from build123d import *

# Parameters (mm, degrees)
F1_DEPTH    = 6.35
F2_T1_DEPTH = 38.1
F2_T3_DEPTH = 33.8463065702
F4_DEPTH    = 6.351


# Not quite as in the source:
# - a fillet or chamfer that OpenCascade refuses, or shapes differently, is made with other operations: its cross-section is extruded or revolved along the edge and cut away or added


with BuildPart() as f1:
    # F0 (on Top) → F1 (new body)
    with BuildSketch(Plane.XY):
        Polygon((-3.1513119073, 592.2723904558), (-22.2013119073, 592.2723904558), (-22.2013119073, 439.8723904558), (-19.0263119073, 439.8723904558), (-19.0263119073, -68.1276095442), (-6.3263119073, -68.1276095442), (-6.3263119073, 439.8723904558), (-3.1513119073, 439.8723904558), align=None)
    extrude(amount=F1_DEPTH)

    # F2: fillet of radius 6.35 on 4 edges, made by hand

    # F2_s2 → F2_t1 (cut)
    with BuildSketch(Plane.XY.offset(-15.875)):
        with BuildLine():
            ThreePointArc((-3.1513119073, 585.9223904558), (-5.0111838468, 590.4125185164), (-9.5013119073, 592.2723904558))
            Line((-9.5013119073, 592.2723904558), (-3.1513119073, 592.2723904558))
            Line((-3.1513119073, 592.2723904558), (-3.1513119073, 585.9223904558))
        make_face()
        with BuildLine():
            ThreePointArc((-15.8513119073, 592.2723904558), (-20.3414399678, 590.4125185164), (-22.2013119073, 585.9223904558))
            Line((-22.2013119073, 585.9223904558), (-22.2013119073, 592.2723904558))
            Line((-22.2013119073, 592.2723904558), (-15.8513119073, 592.2723904558))
        make_face()
    extrude(amount=F2_T1_DEPTH, mode=Mode.SUBTRACT)

    # F2_s4 → F2_t3 (cut)
    with BuildSketch(Plane.XY.offset(-13.7481532851)):
        with BuildLine():
            ThreePointArc((-22.2013119073, 445.3716517699), (-21.3505732213, 442.1966517699), (-19.0263119073, 439.8723904558))
            Line((-19.0263119073, 439.8723904558), (-22.2013119073, 439.8723904558))
            Line((-22.2013119073, 439.8723904558), (-22.2013119073, 445.3716517699))
        make_face()
        with BuildLine():
            ThreePointArc((-6.3263119073, 439.8723904558), (-4.0020505933, 442.1966517699), (-3.1513119073, 445.3716517699))
            Line((-3.1513119073, 445.3716517699), (-3.1513119073, 439.8723904558))
            Line((-3.1513119073, 439.8723904558), (-6.3263119073, 439.8723904558))
        make_face()
    extrude(amount=F2_T3_DEPTH, mode=Mode.SUBTRACT)

    # F3 (on face) → F4 (cut, through all)
    with BuildSketch(Plane(origin=(0, 0, 0), x_dir=(1, 0, 0), z_dir=(0, 0, -1))):
        with BuildLine():
            Line((-16.1688119073, -471.6223904558), (-16.1688119073, -573.2223904558))
            ThreePointArc((-16.1688119073, -573.2223904558), (-12.6763119073, -576.7148904558), (-9.1838119073, -573.2223904558))
            Line((-9.1838119073, -573.2223904558), (-9.1838119073, -471.6223904558))
            ThreePointArc((-9.1838119073, -471.6223904558), (-12.6763119073, -468.1298904558), (-16.1688119073, -471.6223904558))
        make_face()
    extrude(amount=-F4_DEPTH, mode=Mode.SUBTRACT)


solid = f1.part
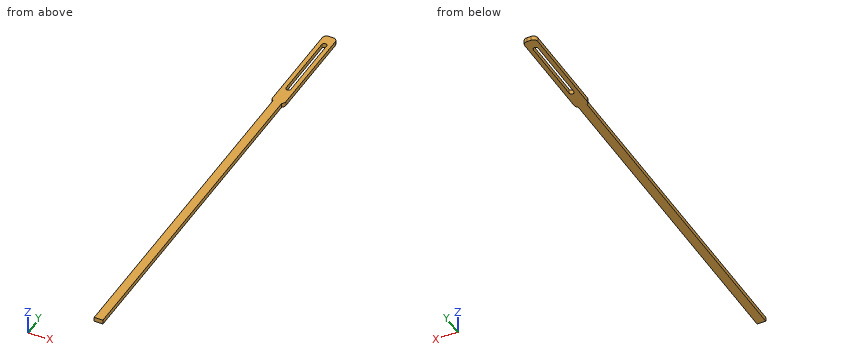
The model under review builds one solid part; all positions refer to its coordinate system, in mm. Give positions to 0.01 mm unless a question says otherwise; leave off trailing zeros. Order: outer loops, then holes, each group sorted by start corner. A loop starts at its lowest first (then second) coordinate and runs counter-clockwise, first axis right, second up. Notation, with made-up numbers: M -33,56 L -6,56 A23 ccw -6,88 Z; hole C -5,33.5 d2. An arc over 180 degrees is marked long. Answer in a Markdown table with one row per item. Add a question column.
1. For pin 1 Ø3 at (y, z) = (89.5, 4) entering from +X, flat-tipped, find the tip position at first contact; note if it passes through.
2. Add section B-B on y = 529.5. State the section outline as (x, z) points.
3. Add section C-C on y = 334. State the section outline as (x, z) points.
4. To check wall thickness, follow line 1 along X through (y, z) = (487, 3.25); line 2 along X through (y, z) = (-27.5, 6.25); line 3 along Y through (x, z) = (-16.5, 6.25). State the ranges of each line that lie inside material, in increasing order.
The answers:
| question | item | result |
|---|---|---|
| 1 | pin 1 | x = -6.33 |
| 2 | outline | M -22.2,0 L -16.17,0 L -16.17,6.35 L -22.2,6.35 Z; M -9.18,0 L -3.15,0 L -3.15,6.35 L -9.18,6.35 Z |
| 3 | outline | M -19.03,0 L -6.33,0 L -6.33,6.35 L -19.03,6.35 Z |
| 4 | line 1 | -22.2 to -16.17, -9.18 to -3.15 |
| 4 | line 2 | -19.03 to -6.33 |
| 4 | line 3 | -68.13 to 592.24 |
